Geometry check sheet. Reference: the model listing, model coordinates, mm. A direction names the side the tool comes from. Give positions to 0.01 mm unless a question says otherwise; leave off trailing zeros. Order: outer loops, then holes, each group sorted by start corner. A loop starts at its lowest first (then second) coordinate and runs counter-clockwise, first axis right, second up. Notation, with made-up numbers: M 53,65 L 72,65 A25 cw 72,97 Z; hole C 87,32 d9. An arc over 180 degrees is marked long. Put each result on its own line as item: value. Start each with the question number.
Q1. Section check C-C on x = 1.5. Record the cut outline in (y, z).
Q2. Go/stop test with flat-tipped pins: pin 1 (1.4 mm diameter, centred on x = -15, y = 15, fed in from +Z); pin 2 (8 mm diameter, centred on x = 4, z = 2.5, fed in from -Y); pin 3 (1 mm diameter, centred on x = 4.5, z = 13.5, fed in from -Y). Record where each tip stops, or that it passes through.
Q3. Section check A-A on z = 11.5. Record the cut outline in (x, y).
Q4. Mould release check, pull along Y, two halves, no side actions. Record for faces 1 (the cylindrical face through (-17.215, 17.199, 7.098)), 2 (the cylindrical face through (-8.63, 8.3, 6.08)), 3 (the flat face through (8, 9, 6)), 4 (the flat face through (-8, 8, 0)): +Y half, -Y half, draft (parallel to the pull), parting line (faces both ways), or undercut.
Q5. Access from +Z, -Z, +X, -X, +Y, -Y to the whole of each face (thin tool, end or side, straight path). Record for faces 5 (the flat face through (-15, -2, 13)), 6 (the flat face through (-16, 8, 14)), 7 (the cylindrical face through (-14, 15.1, 13)).
Q6. Section check B-B on y = -6. Record the cut outline in (x, z), then the cut area to 3 significant figures.
Q7. Material ranges on L1, parallel to Z at x = -11.5, y = 14.5; L2, parallel to X at y = 1, z = 5.75; L3, parallel to Y at x = 15.5, z = 11.5, recorded low to high.
```python
from build123d import *

# Parameters (mm, degrees)
F0_W      = 35
F0_H      = 35
F1_DEPTH  = 12
F3_DEPTH  = 2
F4_R      = 0.79375
F5_DEPTH  = 12.001
F7_DEPTH  = 12.001
F8_R      = 0.75
F9_DEPTH  = 2
F10_R     = 2
F12_DEPTH = 12.001
F13_R     = 1


with BuildPart() as f1:
    # F0 (on Top) → F1 (new body)
    with BuildSketch(Plane.XY):
        Rectangle(F0_W, F0_H)
    extrude(amount=F1_DEPTH)

    # F2 (on face) → F3 (join)
    with BuildSketch(Plane.XY.offset(12)):
        Polygon((17.5, 17.5), (-17.5, 17.5), (-17.5, -17.5), (-15, -17.5), (-15, 15), (17.5, 15), align=None)
    extrude(amount=F3_DEPTH)

    # F4 (on face) → F5 (cut, through all)
    with BuildSketch(Plane.XY.offset(12)):
        with Locations((-9, 9)):
            Circle(F4_R)
    extrude(amount=-F5_DEPTH, mode=Mode.SUBTRACT)

    # F6 (on face) → F7 (cut, through all)
    with BuildSketch(Plane.XY.offset(12)):
        with BuildLine():
            Line((12.5, 9), (-3.20625, 9))
            ThreePointArc((-3.20625, 9), (-4.9032000865, 4.9032000865), (-9, 3.20625))
            Line((-9, 3.20625), (-9, -12.5))
            Line((-9, -12.5), (12.5, -12.5))
            Line((12.5, -12.5), (12.5, 9))
        make_face()
    extrude(amount=-F7_DEPTH, mode=Mode.SUBTRACT)

    # F8 (on face) → F9 (cut, through all)
    with BuildSketch(Plane.XY.offset(14)):
        with Locations((-15, 15)):
            Circle(F8_R)
    extrude(amount=-F9_DEPTH, mode=Mode.SUBTRACT)

    # F10
    f10_edges = [f1.edges().sort_by_distance(p)[0] for p in [
        (-3.20625, 9, 6),
        (-9, 3.20625, 6),
        (12.5, 9, 6),
        (12.5, -12.5, 6),
        (-9, -12.5, 6),
    ]]
    fillet(f10_edges, radius=F10_R)

    # F11 (on face) → F12 (cut, through all)
    with BuildSketch(Plane.XY.offset(12)):
        Polygon((10.5, 9), (-9, -10.5), (-9, -17.5), (17.5, -17.5), (17.5, 9), align=None)
    extrude(amount=-F12_DEPTH, mode=Mode.SUBTRACT)

    # F13
    f13_edges = [f1.edges().sort_by_distance(p)[0] for p in [
        (17.5, 17.5, 7),
        (-17.5, -17.5, 7),
        (-17.5, 17.5, 7),
        (-15, -17.5, 13),
        (17.5, 15, 13),
        (-15, 14.25, 13),
        (-14.25, 15, 13),
        (-9, -17.5, 6),
        (17.5, 9, 6),
    ]]
    fillet(f13_edges, radius=F13_R)


solid = f1.part
```
Results found:
1. outline: M 9,0 L 17.5,0 L 17.5,14 L 15,14 L 15,12 L 9,12 Z
2. pin 1: stops at z = 12
2. pin 2: stops at y = 9
2. pin 3: stops at y = 15
3. outline: M -17.5,-16.5 A1 ccw -16.5,-17.5 L -10,-17.5 A1 ccw -9,-16.5 L -9,1.47 A2 cw -7.51,3.4 A5.79 ccw -3.4,7.51 A2 cw -1.47,9 L 16.5,9 A1 ccw 17.5,10 L 17.5,16.5 A1 ccw 16.5,17.5 L -16.5,17.5 A1 ccw -17.5,16.5 Z; hole C -9,9 d1.59
4. face 1: +Y half
4. face 2: undercut
4. face 3: -Y half
4. face 4: draft
5. face 5: +Z, +X, -Y
5. face 6: +Z, +X, -X, +Y, -Y
5. face 7: +Z, -Y
6. outline: M -17.5,0 L -9,0 L -9,12 L -15,12 L -15,14 L -17.5,14 Z
6. area: 107 mm^2
7. L1: z = 0 to 12
7. L2: x = -17.5 to -9
7. L3: y = 9 to 17.5
